```python
from build123d import *

# Parameters (mm, degrees)
BOSS_EXTRUDE1_DEPTH            = 81.28
SKETCH3_W                      = 76.2
SKETCH3_H                      = 50.292
CUT_EXTRUDE1_DEPTH             = 37.846
SKETCH4_W                      = 40.386
SKETCH4_H                      = 43.18
CUT_EXTRUDE2_DEPTH             = 52.832
FILLET1_R                      = 2.54
FILLET2_R                      = 2.54
FILLET3_R                      = 2.54
FILLET4_R                      = 2.54
SKETCH7_W                      = 16.51
SKETCH7_H                      = 2.54
CUT_EXTRUDE4_REACH             = 54.566
SKETCH8_W                      = 16.51
SKETCH8_H                      = 16.012242806
CUT_EXTRUDE4_DIRECTION_2_DEPTH = 2.54
FILLET5_R                      = 1.27


with BuildPart() as part:
    # Sketch1 → Boss-Extrude1 (new body)
    with BuildSketch(Plane.XY):
        with BuildLine():
            Line((0, 52.9844), (0, 58.0644))
            ThreePointArc((0, 58.0644), (12.7, 70.7644), (0, 83.4644))
            Line((0, 83.4644), (0, 98.7044))
            Line((0, 98.7044), (40.386, 98.7044))
            Line((40.386, 98.7044), (40.386, 25.398729968))
            ThreePointArc((40.386, 25.398729968), (40.827682914, 17.344312358), (42.147434783, 9.386487162))
            ThreePointArc((42.147434783, 9.386487162), (33.688432107, -27.011144777), (0, -43.18))
            Line((0, -43.18), (0, -29.4894))
            ThreePointArc((0, -29.4894), (29.4894, 0), (0, 29.4894))
            Line((0, 29.4894), (0, 52.9844))
        make_face()
    extrude(amount=-BOSS_EXTRUDE1_DEPTH)

    # Sketch3 → Cut-Extrude1 (cut)
    with BuildSketch(Plane.ZY):
        with Locations((-40.64, 71.0184)):
            Rectangle(SKETCH3_W, SKETCH3_H)
    extrude(amount=-CUT_EXTRUDE1_DEPTH, mode=Mode.SUBTRACT)

    # Sketch4 → Cut-Extrude2 (cut)
    with BuildSketch(Plane(origin=(0, 98.7044, 0), x_dir=(1, 0, 0), z_dir=(0, 1, 0))):
        with Locations((20.193, 40.64)):
            Rectangle(SKETCH4_W, SKETCH4_H)
    extrude(amount=-CUT_EXTRUDE2_DEPTH, mode=Mode.SUBTRACT)

    # Fillet1
    fillet1_edges = [part.edges().sort_by_distance(p)[0] for p in [
        (18.923, 45.8724, -78.74),
        (18.923, 45.8724, -2.54),
        (37.846, 45.8724, -10.795),
        (37.846, 45.8724, -70.485),
    ]]
    fillet(fillet1_edges, radius=FILLET1_R)

    # Fillet2
    fillet2_edges = [part.edges().sort_by_distance(p)[0] for p in [
        (37.846, 96.1644, -70.485),
        (37.846, 96.1644, -10.795),
    ]]
    fillet(fillet2_edges, radius=FILLET2_R)

    # Fillet3
    fillet3_edges = [part.edges().sort_by_distance(p)[0] for p in [
        (36.576, 45.8724, -19.05),
        (36.576, 45.8724, -62.23),
    ]]
    fillet(fillet3_edges, radius=FILLET3_R)

    # Fillet4
    fillet4_edges = [part.edges().sort_by_distance(p)[0] for p in [
        (40.386, 98.7044, -71.755),
        (40.386, 98.7044, -9.525),
    ]]
    fillet(fillet4_edges, radius=FILLET4_R)

    # Sketch7 → Cut-Revolve2 (revolve, cut)
    with BuildSketch(Plane.ZY):
        with Locations((-40.64, -41.91)):
            Rectangle(SKETCH7_W, SKETCH7_H)
    revolve(axis=Axis((0, 0, -81.28), (0, 0, 1)), mode=Mode.SUBTRACT)

    # Sketch8 → Cut-Extrude4 (cut, up to next)
    with BuildSketch(Plane(origin=(42.147434783, 9.386487162, 0), x_dir=(0, 0, -1), z_dir=(0.976086957, 0.217380435, 0)), mode=Mode.PRIVATE) as cut_extrude4_sk1:
        with Locations((40.64, 8.006121403)):
            Rectangle(SKETCH8_W, SKETCH8_H)
    cut_extrude4_tool1 = extrude(cut_extrude4_sk1.sketch, amount=-CUT_EXTRUDE4_REACH, mode=Mode.PRIVATE) & part.part
    add(cut_extrude4_tool1.solids().sort_by_distance((40.407061, 17.201158, -40.64))[0], mode=Mode.SUBTRACT)

    # Sketch8 → Cut-Extrude4 direction 2 (cut)
    with BuildSketch(Plane(origin=(42.147434783, 9.386487162, 0), x_dir=(0, 0, -1), z_dir=(0.976086957, 0.217380435, 0))):
        with Locations((40.64, 8.006121403)):
            Rectangle(SKETCH8_W, SKETCH8_H)
    extrude(amount=CUT_EXTRUDE4_DIRECTION_2_DEPTH, mode=Mode.SUBTRACT)

    # Fillet5
    fillet5_edges = [part.edges().sort_by_distance(p)[0] for p in [
        (40.64, 0, -48.895),
        (40.64, 0, -32.385),
    ]]
    fillet(fillet5_edges, radius=FILLET5_R)


solid = part.part
```
Check sheet for the modelled part. Datum: model origin and axes. Units: mm. A direction names the side the tool comes from. Give positions to 0.01 mm unless a question says otherwise; leave off trailing zeros. Loops run counter-clockwise (first coordinate to the right, second up) from the corner with the lowest first, then second, coordinate; pieces in that order, holes last. Notation, with made-up numbers: M 33,36.25 L 82,36.25 A13 cw 82,50.25 Z; hole C 80.25,-20.5 d7. An arc over 180 degrees is marked long. Answer as CSV lines item,"result".
Item 1: Set-up check for faces 1 (the face through (38.4, 46.3, -61.1)), 2 (the face through (40.63, -0.89, -40.54)), 3 (the face through (23, 72, -2.54)), 4 (the face through (40.815, 17.457, -64.861)): record each of +Z, -Z, +X, -X, +Y, -Y from which the full face is reachable in a straight line by a thin tool's end or side.
Reply:
face 1,"+X, -X, +Y"
face 2,"none"
face 3,"-X"
face 4,"+Z, -Z, +X, +Y"
Item 2: Sectioned sample at C-C, the plane z = -69. Enter the section's corners in (x, y), then the cut area to 3 significant figures.
Reply:
outline,"M 0,-43.18 A43.18 ccw 42.15,9.39 A73.66 cw 40.39,25.4 L 40.39,96.16 A2.54 ccw 37.85,98.7 L 0,98.7 L 0,96.16 L 35.31,96.16 A2.54 cw 37.85,93.62 L 37.85,48.41 A2.54 cw 35.31,45.87 L 0,45.87 L 0,29.49 A29.49 cw 0,-29.49 Z"
area,"2,220 mm^2"
Item 3: Sectioned sample at B-B, the plane x = 21.5. State how many separate pieces and enclosed holes the cut face has, then the cut area to 3 significant figures.
Reply:
separate pieces,"2"
enclosed holes,"1"
area,"3,750 mm^2"
Item 4: Scan lines: L1, parallel to Z at x = 9, y = 87.5; L2, parallel to Y at x = 17.5, z = -63; L3, parallel to Y at x = 23.5, z = -16. Record each from-to range of solid material in increasing order.
Reply:
L1,"-81.28 to -78.74, -2.54 to 0"
L2,"-39.47 to -23.74, 23.74 to 45.87, 96.16 to 98.7"
L3,"-36.23 to -17.82, 17.82 to 45.87, 96.16 to 98.7"
Item 5: Draft check along Z on faces 5 (the face through (22, 45, -81.28)), 6 (the face through (39.6, 98, -71.9)), 7 (the face through (42, -4, -48.895)). Enter one of: pulls with the +Z half, pulls with the -Z half, needs draft (parallel to the pull), parting line crosses it, or undercut.
Reply:
face 5,"pulls with the -Z half"
face 6,"needs draft"
face 7,"undercut"
Item 6: Sectioned sample at A-A, the plane y = 68.5. Enter the section's corners in (x, z).
Reply:
outline,"M 12.5,-81.28 L 40.39,-81.28 L 40.39,-62.23 L 37.85,-62.23 L 37.85,-78.74 L 12.5,-78.74 Z; M 12.5,-2.54 L 37.85,-2.54 L 37.85,-19.05 L 40.39,-19.05 L 40.39,0 L 12.5,0 Z"
Item 7: Sectioned sample at D-D, the plane y = 0. Enter the section's corners in (x, z) (3 decimals), then the cut area to 3 significant figures.
Reply:
outline,"M 29.489,-81.28 L 43.18,-81.28 L 43.18,-48.895 L 41.91,-48.895 A1.27 cw 40.64,-47.625 L 40.64,-33.655 A1.27 cw 41.91,-32.385 L 43.18,-32.385 L 43.18,0 L 29.489,0 Z"
area,"1,070 mm^2"
Item 8: Depth check by flat-ended pin: pin 1 Ø3 at (y, z) = (0.5, -15) entering from +X; pin 2 Ø1.5 at (y, z) = (-9.5, -49.5) entering from -X; pin 3 Ø8.5 at (x, z) = (16, -12) entering from -Y. Enter the tip coordinate at first touch or a pass-through.
Reply:
pin 1,"x = 43.18"
pin 2,"x = 27.65"
pin 3,"y = -41.55"
